Geometry check sheet. Reference: the model listing, model coordinates, mm. Face numbers are marked on the shaded views. A direction names the side the tool comes from. Give positions to 0.01 mm unless a question says otherwise; leave off trailing zeros. Write each loop counter-clockwise with the first axis right and the second up, starting at its lowest first coordinate (ties: lowest second). Pieces come first, ordered by that corner, then holes. Notation, with made-up numbers: (75.5, 19.25) - (112.5, 19.25) arc R11 cw to (112.5, 30.25) - close; hole circle Ø8 at (-26.5, -10.75). An arc over 180 degrees is marked (long way). Write item = value, one per line. Start each with the question number.
(1) Depth check by flat-ended pin: pin 1 Ø2.5 at (x, z) = (4.22, -19.71) entering from -Y; pin 2 Ø4 at (x, y) = (3.22, 9) entering from -Z; pin 3 Ø20 at (x, z) = (-9, 8) entering from +Y. Enter the tip coordinate at first touch or a pass-through.
(2) Section check D-D, the plane z = 23.5. Enter the section's corners in (x, y), plus the area to 3 significant figures.
(3) Section check A-A, the plane x = -6. Enter the section's corners in (y, z) (3 decimals), plus the area to 3 significant figures.
(4) Thickness scan on L1, parallel to Z at x = 2.5, y = 14; L2, parallel to Y at x = 3, z = 19.5. Record the ranges inside material, lowest first.
(5) Access from +Z, -Z, +X, -X, +Y, -Y to the whole of each face (thin tool, end or side, straight path). Record for the marked faces 1 and 2.
(6) Section check B-B, the plane y = 33. Enter the section's corners in (x, z).
(7) Section check C-C, the plane z = -10. Enter the section's corners in (x, y), plus the area to 3 significant figures.
```python
from build123d import *

# Parameters (mm, degrees)
EXTRUDE_1_DEPTH     = 3
SKETCH_3_W          = 40
SKETCH_3_H          = 3
EXTRUDE_2_DEPTH     = 39
CUT_EXTRUDE_1_REACH = 76.012
CUT_EXTRUDE_2_REACH = 59.234
SKETCH_5_R          = 1.5
SKETCH_5_R_2        = 11.5
CUT_EXTRUDE_3_REACH = 76.012
SKETCH_6_R          = 1.55


with BuildPart() as part:
    # 草图2 → 凸台-拉伸1 (new body)
    with BuildSketch(Plane(origin=(0, 0, 0), x_dir=(1, 0, 0), z_dir=(0, 1, 0))):
        with BuildLine():
            Line((-26.777777778, 24.707602339), (3.222222222, 24.707602339))
            ThreePointArc((3.222222222, 24.707602339), (6.757756128, 23.243136245), (8.222222222, 19.707602339))
            Line((8.222222222, 19.707602339), (8.222222222, -27.292397661))
            Line((8.222222222, -27.292397661), (-31.777777778, -27.292397661))
            Line((-31.777777778, -27.292397661), (-31.777777778, 19.707602339))
            ThreePointArc((-31.777777778, 19.707602339), (-30.313311684, 23.243136245), (-26.777777778, 24.707602339))
        make_face()
    extrude(amount=EXTRUDE_1_DEPTH)

    # 草图3 → 凸台-拉伸2 (add)
    with BuildSketch(Plane(origin=(0, 3, 0), x_dir=(1, 0, 0), z_dir=(0, 1, 0))):
        with Locations((-11.777777778, -25.792397661)):
            Rectangle(SKETCH_3_W, SKETCH_3_H)
    extrude(amount=EXTRUDE_2_DEPTH)

    # 草图4 → 切除-拉伸1 (cut, up to next)
    with BuildSketch(Plane.XY.offset(27.292397661), mode=Mode.PRIVATE) as cut_extrude_1_sk1:
        with BuildLine():
            Line((-31.777777778, 37), (-31.777777778, 42))
            Line((-31.777777778, 42), (-26.777777778, 42))
            ThreePointArc((-26.777777778, 42), (-30.313311684, 40.535533906), (-31.777777778, 37))
        make_face()
    cut_extrude_1_tool1 = extrude(cut_extrude_1_sk1.sketch, amount=-CUT_EXTRUDE_1_REACH, mode=Mode.PRIVATE) & part.part
    # 草图4 → 切除-拉伸1 (cut, up to next)
    with BuildSketch(Plane.XY.offset(27.292397661), mode=Mode.PRIVATE) as cut_extrude_1_sk2:
        with BuildLine():
            Line((3.222222222, 42), (8.222222222, 42))
            Line((8.222222222, 42), (8.222222222, 37))
            ThreePointArc((8.222222222, 37), (6.757756128, 40.535533906), (3.222222222, 42))
        make_face()
    cut_extrude_1_tool2 = extrude(cut_extrude_1_sk2.sketch, amount=-CUT_EXTRUDE_1_REACH, mode=Mode.PRIVATE) & part.part
    add(cut_extrude_1_tool1.solids().sort_by_distance((-30.660938, 40.88316, 27.292398))[0], mode=Mode.SUBTRACT)
    add(cut_extrude_1_tool2.solids().sort_by_distance((7.105383, 40.88316, 27.292398))[0], mode=Mode.SUBTRACT)

    # 草图5 → 切除-拉伸2 (cut, up to next)
    with BuildSketch(Plane(origin=(0, 3, 0), x_dir=(1, 0, 0), z_dir=(0, 1, 0)), mode=Mode.PRIVATE) as cut_extrude_2_sk1:
        with Locations(Location((-26.777777778, 19.707602339, 0), (0, 0, 270))):
            Circle(SKETCH_5_R)
    cut_extrude_2_tool1 = extrude(cut_extrude_2_sk1.sketch, amount=-CUT_EXTRUDE_2_REACH, mode=Mode.PRIVATE) & part.part
    # 草图5 → 切除-拉伸2 (cut, up to next)
    with BuildSketch(Plane(origin=(0, 3, 0), x_dir=(1, 0, 0), z_dir=(0, 1, 0)), mode=Mode.PRIVATE) as cut_extrude_2_sk2:
        with Locations(Location((4.222222222, 19.707602339, 0), (0, 0, 270))):
            Circle(SKETCH_5_R)
    cut_extrude_2_tool2 = extrude(cut_extrude_2_sk2.sketch, amount=-CUT_EXTRUDE_2_REACH, mode=Mode.PRIVATE) & part.part
    # 草图5 → 切除-拉伸2 (cut, up to next)
    with BuildSketch(Plane(origin=(0, 3, 0), x_dir=(1, 0, 0), z_dir=(0, 1, 0)), mode=Mode.PRIVATE) as cut_extrude_2_sk3:
        with Locations(Location((-26.777777778, -11.292397661, 0), (0, 0, 270))):
            Circle(SKETCH_5_R)
    cut_extrude_2_tool3 = extrude(cut_extrude_2_sk3.sketch, amount=-CUT_EXTRUDE_2_REACH, mode=Mode.PRIVATE) & part.part
    # 草图5 → 切除-拉伸2 (cut, up to next)
    with BuildSketch(Plane(origin=(0, 3, 0), x_dir=(1, 0, 0), z_dir=(0, 1, 0)), mode=Mode.PRIVATE) as cut_extrude_2_sk4:
        with Locations(Location((4.222222222, -11.292397661, 0), (0, 0, 270))):
            Circle(SKETCH_5_R)
    cut_extrude_2_tool4 = extrude(cut_extrude_2_sk4.sketch, amount=-CUT_EXTRUDE_2_REACH, mode=Mode.PRIVATE) & part.part
    # 草图5 → 切除-拉伸2 (cut, up to next)
    with BuildSketch(Plane(origin=(0, 3, 0), x_dir=(1, 0, 0), z_dir=(0, 1, 0)), mode=Mode.PRIVATE) as cut_extrude_2_sk5:
        with Locations(Location((-11.277777778, 4.207602339, 0), (0, 0, 270))):
            Circle(SKETCH_5_R_2)
    cut_extrude_2_tool5 = extrude(cut_extrude_2_sk5.sketch, amount=-CUT_EXTRUDE_2_REACH, mode=Mode.PRIVATE) & part.part
    add(cut_extrude_2_tool1.solids().sort_by_distance((-26.777778, 3, -19.707602))[0], mode=Mode.SUBTRACT)
    add(cut_extrude_2_tool2.solids().sort_by_distance((4.222222, 3, -19.707602))[0], mode=Mode.SUBTRACT)
    add(cut_extrude_2_tool3.solids().sort_by_distance((-26.777778, 3, 11.292398))[0], mode=Mode.SUBTRACT)
    add(cut_extrude_2_tool4.solids().sort_by_distance((4.222222, 3, 11.292398))[0], mode=Mode.SUBTRACT)
    add(cut_extrude_2_tool5.solids().sort_by_distance((-11.277778, 3, -4.207602))[0], mode=Mode.SUBTRACT)

    # 草图6 → 切除-拉伸3 (cut, up to next)
    with BuildSketch(Plane.XY.offset(27.292397661), mode=Mode.PRIVATE) as cut_extrude_3_sk1:
        with Locations((-27.59761171, 9)):
            Circle(SKETCH_6_R)
    cut_extrude_3_tool1 = extrude(cut_extrude_3_sk1.sketch, amount=-CUT_EXTRUDE_3_REACH, mode=Mode.PRIVATE) & part.part
    # 草图6 → 切除-拉伸3 (cut, up to next)
    with BuildSketch(Plane.XY.offset(27.292397661), mode=Mode.PRIVATE) as cut_extrude_3_sk2:
        with Locations((-27.59761171, 33)):
            Circle(SKETCH_6_R)
    cut_extrude_3_tool2 = extrude(cut_extrude_3_sk2.sketch, amount=-CUT_EXTRUDE_3_REACH, mode=Mode.PRIVATE) & part.part
    # 草图6 → 切除-拉伸3 (cut, up to next)
    with BuildSketch(Plane.XY.offset(27.292397661), mode=Mode.PRIVATE) as cut_extrude_3_sk3:
        with Locations((3.222222222, 9)):
            Circle(SKETCH_6_R)
    cut_extrude_3_tool3 = extrude(cut_extrude_3_sk3.sketch, amount=-CUT_EXTRUDE_3_REACH, mode=Mode.PRIVATE) & part.part
    # 草图6 → 切除-拉伸3 (cut, up to next)
    with BuildSketch(Plane.XY.offset(27.292397661), mode=Mode.PRIVATE) as cut_extrude_3_sk4:
        with Locations((3.222222222, 33)):
            Circle(SKETCH_6_R)
    cut_extrude_3_tool4 = extrude(cut_extrude_3_sk4.sketch, amount=-CUT_EXTRUDE_3_REACH, mode=Mode.PRIVATE) & part.part
    add(cut_extrude_3_tool1.solids().sort_by_distance((-27.597612, 9, 27.292398))[0], mode=Mode.SUBTRACT)
    add(cut_extrude_3_tool2.solids().sort_by_distance((-27.597612, 33, 27.292398))[0], mode=Mode.SUBTRACT)
    add(cut_extrude_3_tool3.solids().sort_by_distance((3.222222, 9, 27.292398))[0], mode=Mode.SUBTRACT)
    add(cut_extrude_3_tool4.solids().sort_by_distance((3.222222, 33, 27.292398))[0], mode=Mode.SUBTRACT)


solid = part.part
```
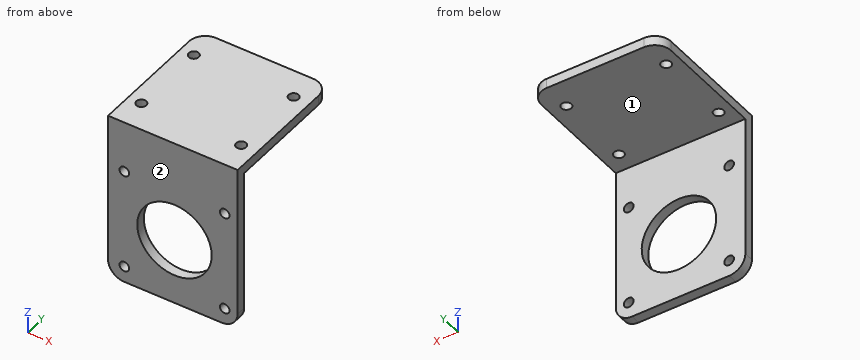
Model answer:
q1.pin_1 = through
q1.pin_2 = 24.29
q1.pin_3 = 3
q2.outline = (-31.78, 0) - (8.22, 0) - (8.22, 3) - (-31.78, 3) - close
q2.area = 120 mm²
q3.outline = (0, -24.708) - (3, -24.708) - (3, -14.425) - (0, -14.425) - close; (0, 6.01) - (3, 6.01) - (3, 24.292) - (42, 24.292) - (42, 27.292) - (0, 27.292) - close
q3.area = 212 mm²
q4.L1 = 24.29 to 27.29
q4.L2 = 0 to 3
q5.face_1 = -Z, +X, -X, +Y
q5.face_2 = +Z, -Z, +X, -X, -Y
q6.outline = (-31.78, 24.29) - (-29.15, 24.29) - (-29.15, 27.29) - (-31.78, 27.29) - close; (-26.05, 24.29) - (1.67, 24.29) - (1.67, 27.29) - (-26.05, 27.29) - close; (4.77, 24.29) - (8.22, 24.29) - (8.22, 27.29) - (4.77, 27.29) - close
q7.outline = (-31.78, 0) - (-21.21, 0) - (-21.21, 3) - (-31.78, 3) - close; (-1.34, 0) - (8.22, 0) - (8.22, 3) - (-1.34, 3) - close
q7.area = 60.4 mm²
